```python
from build123d import *

# Parameters (mm, degrees)
F_5_16_CLEARANCE_HOLE1_D         = 8.4328
CIRPATTERN1_COUNT                = 12
F_1_2_0_5_DIAMETER_HOLE1_D       = 12.7
F_1_1_5_DIAMETER_HOLE1_D         = 38.1
F_1_1_5_DIAMETER_HOLE1_DEPTH     = 19.05
CIRPATTERN2_COUNT                = 6
CIRPATTERN3_COUNT                = 2
F_1_8_0_125_DIAMETER_HOLE1_D     = 3.175
F_1_8_0_125_DIAMETER_HOLE1_DEPTH = 6.35
F_1_8_0_125_DIAMETER_HOLE1_TIP   = 0.953866233


with BuildPart() as part:
    # Sketch1 → Revolve1 (revolve)
    with BuildSketch(Plane.XY, mode=Mode.PRIVATE) as revolve1_sk:
        Polygon((-88.9, 0), (-88.9, 41.275), (-50.8, 41.275), (-31.75, 60.325), (0, 60.325), (0, 34.925), (-31.75, 34.925), (-31.75, 22.225), (-50.8, 22.225), (-50.8, 3.175), (-52.3875, 3.175), (-52.3875, 5.715), (-55.9435, 5.715), (-55.9435, 3.175), (-57.15, 3.175), (-57.15, 0), align=None)
    revolve(revolve1_sk.sketch.rotate(Axis((0, 0, 0), (0, 1, 0)), 270), axis=Axis((0, 0, 0), (0, 1, 0)))

    # 5/16 Clearance Hole1 (through all)
    with Locations(Plane(origin=(0, 41.275, 0), x_dir=(1, 0, 0), z_dir=(0, 1, 0))):
        with Locations((-73.603547963, -19.722011237)):
            f_5_16_clearance_hole1 = Hole(F_5_16_CLEARANCE_HOLE1_D / 2)

    # CirPattern1: 5/16 Clearance Hole1 ×12 about axis
    cirpattern1_axis = Axis((0, 0, 0), (0, 1, 0))
    for i in range(1, CIRPATTERN1_COUNT):
        add(f_5_16_clearance_hole1.rotate(cirpattern1_axis, i * 360 / CIRPATTERN1_COUNT), mode=Mode.SUBTRACT)

    # 1/2 (0.5) Diameter Hole1 (through all)
    with Locations(Plane(origin=(0, 60.325, 0), x_dir=(1, 0, 0), z_dir=(0, 1, 0))):
        with Locations((0, 0)):
            Hole(F_1_2_0_5_DIAMETER_HOLE1_D / 2)

    # Sketch11 → 1/2 NPT Tapped Hole1 (revolve, cut)
    with BuildSketch(Plane(origin=(41.275, 50.8, 0), x_dir=(-0.707106781186546, 0.707106781186549, 0), z_dir=(0, 0, 1))):
        Polygon((0, 0), (0, 127.968649725), (8.9281, 127.968649725), (8.9281, 13.462), (9.479726792, 13.462), (9.8827971, 0), align=None)
    revolve(axis=Axis((45.765128061, 55.290128061, 0), (-0.707106781186549, -0.707106781186546, 0)), mode=Mode.SUBTRACT)

    # 1 (1.5) Diameter Hole1
    with Locations(Plane(origin=(0, 60.325, 0), x_dir=(1, 0, 0), z_dir=(0, 1, 0))):
        with Locations((-23.8125, -41.244459855)):
            f_1_1_5_diameter_hole1 = Hole(F_1_1_5_DIAMETER_HOLE1_D / 2, depth=F_1_1_5_DIAMETER_HOLE1_DEPTH)

    # Sketch19 → 3/8 NPT Tapped Hole1 (revolve, cut)
    with BuildSketch(Plane(origin=(-23.8125, 41.275, 41.244459855), x_dir=(0, 0, 1), z_dir=(1, 0, 0))):
        Polygon((0, 0), (0, 26.640582582), (7.1374, 22.352), (7.1374, 10.414), (7.653732494, 10.414), (7.9655416, 0), align=None)
    f_3_8_npt_tapped_hole1 = revolve(axis=Axis((-23.8125, 47.625, 41.244459855), (0, -1, 0)), mode=Mode.SUBTRACT)

    # Sketch21 → 1/4 (0.25) Diameter Hole1 (revolve, cut)
    with BuildSketch(Plane(origin=(21.997045256, 60.325, -12.7), x_dir=(0, 0, 1), z_dir=(1, 0, 0))):
        Polygon((0, 0), (0, 17.782732465), (3.175, 15.875), (3.175, 0), align=None)
    f_1_4_0_25_diameter_hole1 = revolve(axis=Axis((21.997045256, 66.675, -12.7), (0, -1, 0)), mode=Mode.SUBTRACT)

    # CirPattern2: 1/4 (0.25) Diameter Hole1 ×6 about axis
    cirpattern2_axis = Axis((0, 0, 0), (0, 1, 0))
    for i in range(1, CIRPATTERN2_COUNT):
        add(f_1_4_0_25_diameter_hole1.rotate(cirpattern2_axis, i * 360 / CIRPATTERN2_COUNT), mode=Mode.SUBTRACT)

    # CirPattern3: 1 (1.5) Diameter Hole1, 3/8 NPT Tapped Hole1 ×2 about axis
    cirpattern3_axis = Axis((0, 0, 0), (0, 1, 0))
    add([f_1_1_5_diameter_hole1.rotate(cirpattern3_axis, i * 360 / CIRPATTERN3_COUNT) for i in range(1, CIRPATTERN3_COUNT)], mode=Mode.SUBTRACT)
    add([f_3_8_npt_tapped_hole1.rotate(cirpattern3_axis, i * 360 / CIRPATTERN3_COUNT) for i in range(1, CIRPATTERN3_COUNT)], mode=Mode.SUBTRACT)

    # 1/8 (0.125) Diameter Hole1
    with Locations(Plane(origin=(0, 22.225, 0), x_dir=(-1, 0, 0), z_dir=(0, -1, 0))):
        with Locations((0, 44.45)):
            Hole(F_1_8_0_125_DIAMETER_HOLE1_D / 2, depth=F_1_8_0_125_DIAMETER_HOLE1_DEPTH)
            with Locations((0, 0, -(F_1_8_0_125_DIAMETER_HOLE1_DEPTH + F_1_8_0_125_DIAMETER_HOLE1_TIP / 2))):  # 118° drill point
                Cone(0, F_1_8_0_125_DIAMETER_HOLE1_D / 2, F_1_8_0_125_DIAMETER_HOLE1_TIP, mode=Mode.SUBTRACT)


solid = part.part
```
Input: part model. Units: mm. Frame: model coordinates. A direction names the side the tool comes from. Give positions to 0.01 mm unless a question says otherwise; leave off trailing zeros.
1. Mould query, pull axis Y, two halves, no side actions, for faces 4 (the conical face through (-31.6, 55.2, -19)), 5 (the conical face through (37.474, 45.216, -9.602)), 6 (the cylindrical face through (-0.14, 52.5, 22.23)). Classes: released by +Y, released by -Y, zero draft, split by the parting line, or undercut.
Derived:
face 4: released by +Y
face 5: undercut
face 6: zero draft
2. Reachability of faces 1 (the cylindrical face through (-2.513, 1.565, 57.095)), 2 (the cylindrical face through (55.5, 20.35, -49.99)), 3 (the cylindrical face through (-14.646, 48.55, 24.545)) from +Z, -Z, +X, -X, +Y, -Y: full face, straight path, thin tool, end or side. Return the list, or none.
Derived:
face 1: -Y
face 2: +Y, -Y
face 3: +Y
3. Section A-A on y = 25. Give the number of separate pieces and of enclosed holes in the cut face, and give its area (3 significant figures).
Derived:
separate pieces: 1
enclosed holes: 16
area: 20,700 mm2
4. Pin query (flat end, axial travel): pin 1 (8.5 mm diameter, centred on x = -22, z = 12.7, fed in from -Y) (3 decimals); pin 2 (6 mm diameter, centred on x = 40.5, z = 63, fed in from +Y) (3 decimals); pin 3 (5 mm diameter, centred on x = 0, z = -44.45, fed in from +Y) (3 decimals); pin 4 (7.5 mm diameter, centred on x = 22, z = -12.7, fed in from +Y) (3 decimals). Return the tip coordinate at first contact, or that it passes through.
Derived:
pin 1: stops at y = 34.925
pin 2: stops at y = 41.275
pin 3: stops at y = 50.125
pin 4: stops at y = 60.325
5. Material intervals for L1, parallel to Z at x = -72, y = 13; L2, parallel to Z at x = -1, y = 17; L3, parallel to X at y = 1, z = 0, sorted ascending.
Derived:
L1: z = -52.15 to -23.62, -15.82 to 15.82, 23.62 to 52.15
L2: z = -88.89 to -50.79, 50.79 to 88.89
L3: x = -88.9 to -57.15, 57.15 to 88.9
